```python
from build123d import *

# Parameters (mm, degrees)
CHAMFER1_SIZE      = 1
SKETCH2_W          = 8.626605672
SKETCH2_H          = 1.786618514
CUT_EXTRUDE1_DEPTH = 2


with BuildPart() as part:
    # Sketch1 → Revolve1 (revolve)
    with BuildSketch(Plane.XY):
        Polygon((0, 3.5), (2, 3.5), (2, 0), (3.85, 0), (3.85, 1), (2.85, 1), (2.85, 5), (0, 5), align=None)
    revolve(axis=Axis((0, 3.5, 0), (0, -1, 0)))

    # Chamfer1
    chamfer1_edges = [part.edges().sort_by_distance(p)[0] for p in [
        (-2.85, 5, 0),
    ]]
    chamfer(chamfer1_edges, length=CHAMFER1_SIZE)

    # Sketch2 → Cut-Extrude1 (cut, through all)
    with BuildSketch(Plane(origin=(0, 1, 0), x_dir=(1, 0, 0), z_dir=(0, 1, 0))):
        with Locations((1.724867015, -3.743309257)):
            Rectangle(SKETCH2_W, SKETCH2_H)
    extrude(amount=-CUT_EXTRUDE1_DEPTH, mode=Mode.SUBTRACT)


solid = part.part
```
Check sheet for the modelled part. Datum: model origin and axes. Units: mm. A direction names the side the tool comes from. Coordinates: 2 decimals unless noted, no trailing zeros. Loops run counter-clockwise (first coordinate to the right, second up) from the corner with the lowest first, then second, coordinate; pieces in that order, holes last.
1) Sectioned sample at C-C (y = 4.2). Record the boundary of the cut face in (x, z).
2) Gauge pin test, flat ends, axial feed: pin 1 (2 mm diameter, centred on y = 2.5, z = -2.5, fed in from -X); pin 2 (2 mm diameter, centred on x = -1, y = 2.5, fed in from -Z). Record the tip position at first contact, or that the pin passes through.
3) Sectioned sample at B-B (y = 1.2). Record the boundary of the cut face in (x, z).
4) Sectioned sample at A-A (z = 0). Record the boundary of the cut face in (x, y), and give its area (3 significant figures).
5) Material ranges on probe 1 along Z at (x, y) = (0, 1.7); probe 2 along Z at (x, y) = (0, 0.7); probe 3 along Y at (x, z) = (1.5, -3), recorded low to high.
6) Release check for a two-part mould opening along X. For faces 1 (the face through (-1, 1, -3)), 2 (the face through (0, 3.5, 0)), 3 (the face through (-0.13, 0.507, -3.848)) record: released by +X, released by -X, zero draft, split by the parting line, or undercut.
7) Sectioned sample at D-D (y = 0.7). Record the boundary of the cut face in (x, z).
8) Access from +Z, -Z, +X, -X, +Y, -Y to the whole of each face (thin tool, end or side, straight path). Record for faces 4 (the face through (-2.262, 2.521, -1.734)), 5 (the face through (0, 0.5, 2.85)), 6 (the face through (0, 2, -2)).
Check sheet entries:
1. outline: circle Ø5.3 at (0, 0)
2. pin 1: stops at x = -2.42
2. pin 2: stops at z = -2.85
3. outline: circle Ø5.7 at (0, 0); hole circle Ø4 at (0, 0)
4. outline: (-3.85, 0) - (-2, 0) - (-2, 3.5) - (2, 3.5) - (2, 0) - (3.85, 0) - (3.85, 1) - (2.85, 1) - (2.85, 4) - (1.85, 5) - (-1.85, 5) - (-2.85, 4) - (-2.85, 1) - (-3.85, 1) - close
4. area: 15.5 mm2
5. probe 1: z = -2.85 to -2, 2 to 2.85
5. probe 2: z = -3.85 to -2, 2 to 2.85
5. probe 3: y = 0 to 1
6. face 1: zero draft
6. face 2: undercut
6. face 3: split by the parting line
7. outline: (-2.59, 2.85) arc R3.85 ccw (long way) to (2.59, 2.85) - close; hole circle Ø4 at (0, 0)
8. face 4: +Y
8. face 5: +Z, +X, -X, +Y, -Y
8. face 6: -Y
